Autodesk Inventor part; units mm, degrees
ref_plane "YZ Plane" through (0, 0, 0) normal (1, 0, 0) x (0, 1, 0)
ref_plane "XZ Plane" through (0, 0, 0) normal (0, 1, 0) x (-1, 0, 0)
ref_plane "XY Plane" through (0, 0, 0) normal (0, 0, 1) x (1, 0, 0)
sketch "Эскиз1" plane through (0, 0, 0) normal (0, 1, 0) x (-1, 0, 0)
  line L0 (0, 0) -> (40, 0)
  line L1 (40, 0) -> (40, 60)
  line L2 (40, 60) -> (0, 60)
  line L3 (0, 60) -> (0, 0)
  dimension "d0" = 60
  dimension "d1" = 40
extrude "Выдавливание1" add sketch "Эскиз1" along normal blind 190
sketch "Эскиз2" plane through (0, 190, 0) normal (0, 1, 0) x (1, 0, 0)
  line L0 (-35, -5) -> (-5, -5)
  line L1 (-5, -5) -> (-5, -55)
  line L2 (-5, -55) -> (-35, -55)
  line L3 (-35, -55) -> (-35, -5)
  line L4 (-40, 0) -> (-40, -60)
  line L5 (0, -60) -> (0, 0)
  line L6 (0, 0) -> (-40, 0)
  line L7 (-40, -60) -> (0, -60)
  dimension "d4" = 5
  dimension "d5" = 5
  dimension "d6" = 5
  dimension "d7" = 5
extrude "Выдавливание2" cut sketch "Эскиз2" against normal through all contours L0 L1 L2 L3
sketch "Эскиз3" plane through (-40, 0, 60) normal (0, 0, 1) x (1, 0, 0)
  point P0 (40, 0)
sketch "Эскиз5" plane through (0, 190, 0) normal (0, 1, 0) x (1, 0, 0)
  line L0 (-5, -5) -> (-5, -55)
  line L1 (-5, -55) -> (-35, -55)
  line L2 (-35, -55) -> (-35, -5)
  line L3 (-35, -5) -> (-5, -5)
  line L4 (-40, 0) -> (-40, -60)
  line L5 (-40, -60) -> (0, -60)
  line L6 (0, -60) -> (0, 0)
  line L7 (0, 0) -> (-40, 0)
extrude "Выдавливание4" cut sketch "Эскиз5" against normal blind 100
equation "\"d5\" = d4"
equation "\"d6\" = d4"
equation "\"d7\" = d4"
properties part number "БРУС"
CAD build for the part. Positions are in the model's coordinates, mm. A direction names the side the tool comes from. Round coordinates to 2 decimals unless told otherwise and drop trailing zeros. Order: outer loops, then holes, each group sorted by start corner. A loop starts at its lowest first (then second) coordinate and runs counter-clockwise, first axis right, second up.
Item 1: Probe line 1 along Z through (x, y) = (-30.5, 5); line 2 along X through (y, z) = (5.5, 48). List the from-to ranges inside material, lowest first.
Item 2: Saw through at A-A on x = -25. Write the cut outline in (y, z).
Item 3: Mould opens along X. For faces 3 (the face through (-20, 44, 0)), 4 (the face through (-40, 44, 30)), 5 (the face through (-20, 46, 5)) say: pulls with the +X half, pulls with the -X half, needs draft (parallel to the pull), parting line crosses it, or undercut.
Item 4: Saw through at B-B on z = 38.5. Write the cut outline in (x, y).
Item 5: Tool access for faces 1 (the face through (-38, 90, 30)), 2 (the face through (-20, 46, 55)): list every direction of +Z, -Z, +X, -X, +Y, -Y with a clear straight run to the whole face (end or side of a thin tool).
Item 6: Pin check, flat tip, straight feed: pin 1 (1 mm diameter, centred on x = -4.5, y = 32.5, fed in from -Z). Stop position of the tip, or through.
Item 7: Saw through at C-C on y = 63.5. Write the cut outline in (x, z), then the cut area to 3 significant figures.
Reported:
1. line 1: z = 0 to 5, 55 to 60
1. line 2: x = -40 to -35, -5 to 0
2. outline: (0, 0) - (90, 0) - (90, 5) - (0, 5) - close; (0, 55) - (90, 55) - (90, 60) - (0, 60) - close
3. face 3: needs draft
3. face 4: pulls with the -X half
3. face 5: undercut
4. outline: (-40, 0) - (-35, 0) - (-35, 90) - (-40, 90) - close; (-5, 0) - (0, 0) - (0, 90) - (-5, 90) - close
5. face 1: +Z, -Z, +X, -X, +Y
5. face 2: +Y, -Y
6. pin 1: stops at z = 0
7. outline: (-40, 0) - (0, 0) - (0, 60) - (-40, 60) - close; hole (-35, 5) - (-5, 5) - (-5, 55) - (-35, 55) - close
7. area: 900 mm2
